The figure shows three views and two pictorial views of one solid part (mm, origin at its lowest corner). Answer the questions. A direction names the side the tool comes from. Round coordinates to 2 decimals unless told otherwise and drop trailing zeros. Order: outer loops, then holes, each group sorted by start corner. A loop starts at its lowest first (then second) coordinate and runs counter-clockwise, first axis right, second up. Notation, with made-up numbers: (43, -34) - (95, -34) arc R27 ccw to (95, -5) - close; hole circle Ø7 at (-26, 7.5). An arc over 180 degrees is marked (long way). Use CSV: the item, a comma, the result in double quotes. Start each with the question number.
Item 1: Find section A-A, the plane y = 12. Give the vertices of the cut face in (x, z) (3 decimals), plus the area to 3 significant figures.
Item 2: Flat-ended cylindrical pins translate along their axes: P1, Ø3, axis at x = 12, y = 12, coming from the +Z side; P2, Ø1, axis at x = 8, y = 19, coming from the +Z side; P3, Ø1.5, axis at x = 12.5, z = 12.5, coming from the -Y side; P4, Ø1, axis at x = 4, y = 18.5, coming from the -Z side. Find the tip coordinate at first contact, or state that the pin passes through.
Item 3: Find section C-C, the plane x = 22. Give the vertices of the cut face in (y, z) (3 decimals).
Item 4: Determine the mould class of the marked faces 1, 2, 3 and 4 for opening direction Y: +Y half, -Y half, draft (parallel to the pull), parting line (faces both ways), or undercut.
Item 5: Find section D-D, the plane y = 7.5. Give the vertices of the cut face in (x, z).
Item 6: For the marked faces 5, 6 and 7, determine the directions among +Z, -Z, +X, -X, +Y, -Y from which every point of the face is accessible in a straight line to the end or side of a thin tool.
Item 7: Straight lines are drawn through the part: line 1 along Y through (x, z) = (12, 2.5) (3 decimals); line 2 along Z through (x, y) = (14, 11.5). For each, find the intervals that lie inside material, in ascending order. Write a range as [from, to].
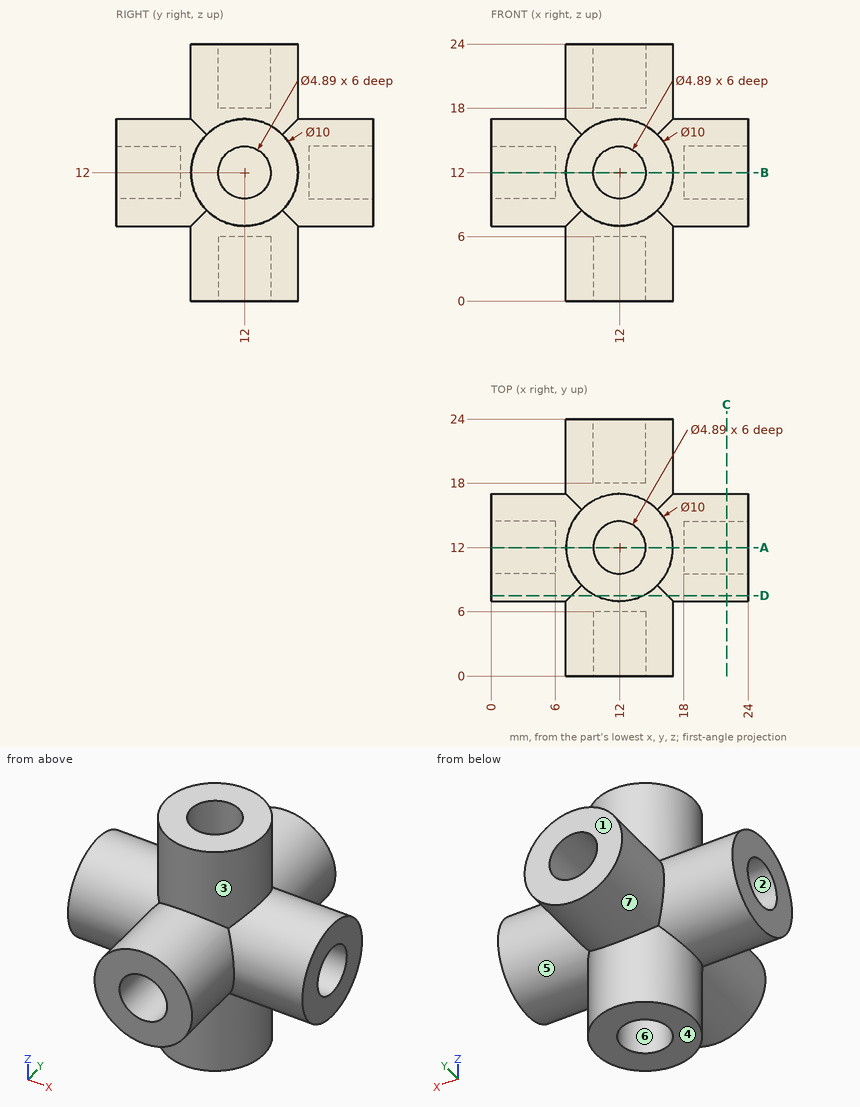
Worked out:
1,outline,"(0, 7) - (7, 7) - (7, 0) - (9.555, 0) - (9.555, 6) - (14.445, 6) - (14.445, 0) - (17, 0) - (17, 7) - (24, 7) - (24, 9.555) - (18, 9.555) - (18, 14.445) - (24, 14.445) - (24, 17) - (17, 17) - (17, 24) - (14.445, 24) - (14.445, 18) - (9.555, 18) - (9.555, 24) - (7, 24) - (7, 17) - (0, 17) - (0, 14.445) - (6, 14.445) - (6, 9.555) - (0, 9.555) - close"
1,area,"263 mm²"
2,P1,"stops at z = 18"
2,P2,"stops at z = 15.57"
2,P3,"stops at y = 6"
2,P4,"passes through"
3,outline,"circle Ø10 at (12, 12); hole circle Ø4.89 at (12, 12)"
4,face 1,"+Y half"
4,face 2,"undercut"
4,face 3,"parting line"
4,face 4,"draft"
5,outline,"(0, 9.82) - (7.5, 9.82) arc R5 ccw to (9.82, 7.5) - (9.82, 0) - (14.18, 0) - (14.18, 7.5) arc R5 ccw to (16.5, 9.82) - (24, 9.82) - (24, 14.18) - (16.5, 14.18) arc R5 ccw to (14.18, 16.5) - (14.18, 24) - (9.82, 24) - (9.82, 16.5) arc R5 ccw to (7.5, 14.18) - (0, 14.18) - close"
6,face 5,"+X"
6,face 6,"-Z"
6,face 7,"+Y"
7,line 1,"y = [7, 9.555], [14.445, 17]"
7,line 2,"z = [6, 18]"
